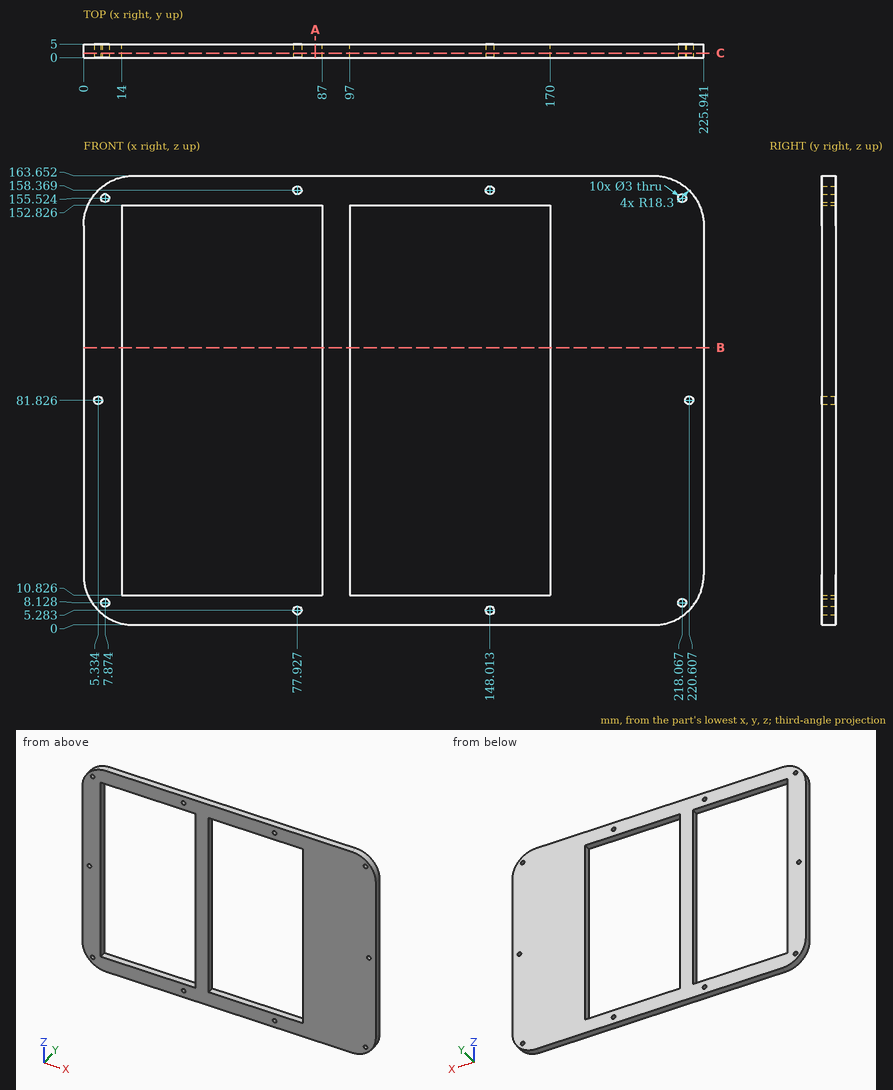
For this review, use the dimensioned drawing (mm, ordinates from the lowest corner) and the shaded views. Give positions to 0.01 mm unless a question says otherwise; leave off trailing zeros. Order: outer loops, then holes, each group sorted by start corner. A loop starts at its lowest first (then second) coordinate and runs counter-clockwise, first axis right, second up. Notation, with made-up numbers: M 45,-24.5 L 76,-24.5 A17 ccw 76,-16.5 Z; hole C 40,39.5 d1. An arc over 180 degrees is marked long. Use one line per item in the form item = value. Start each with the question number.
Item 1: To check wall thickness, follow line 1 along X through (y, z) = (0.45, 81.5); line 2 along X through (y, z) = (3.15, 19); line 3 along Z through (x, y) = (118.5, 3.2). State the ranges of each line that lie inside material, in increasing order. Write a range as from..to.
Item 2: We need section B-B on z = 101. Give the boundary of the cut face in (x, y).
Item 3: We need section A-A on x = 84.5. Give the boundary of the cut face in (y, z), plus the area to 3 significant figures.
Item 4: We need section C-C on y = 1.65. Give the number of separate pieces and of enclosed holes in the cut face, plus the area to 3 significant figures.
Item 5: Insertion check: pin 1 Ø2.5 at (x, z) = (5.33, 81.83) entering from -Y. The pin has a flat end and moves straight along its axis. Give the tip position at first contact, or say it passes through.
Completed:
q1.line_1 = 0..3.87, 6.8..14, 87..97, 170..219.14, 222.07..225.94
q1.line_2 = 0..14, 87..97, 170..225.94
q1.line_3 = 0..10.83, 152.83..163.65
q2.outline = M 0,0 L 14,0 L 14,5 L 0,5 Z; M 87,0 L 97,0 L 97,5 L 87,5 Z; M 170,0 L 225.94,0 L 225.94,5 L 170,5 Z
q3.outline = M 0,0 L 5,0 L 5,10.83 L 0,10.83 Z; M 0,152.83 L 5,152.83 L 5,163.65 L 0,163.65 Z
q3.area = 108 mm²
q4.separate_pieces = 1
q4.enclosed_holes = 12
q4.area = 15,900 mm²
q5.pin_1 = through
